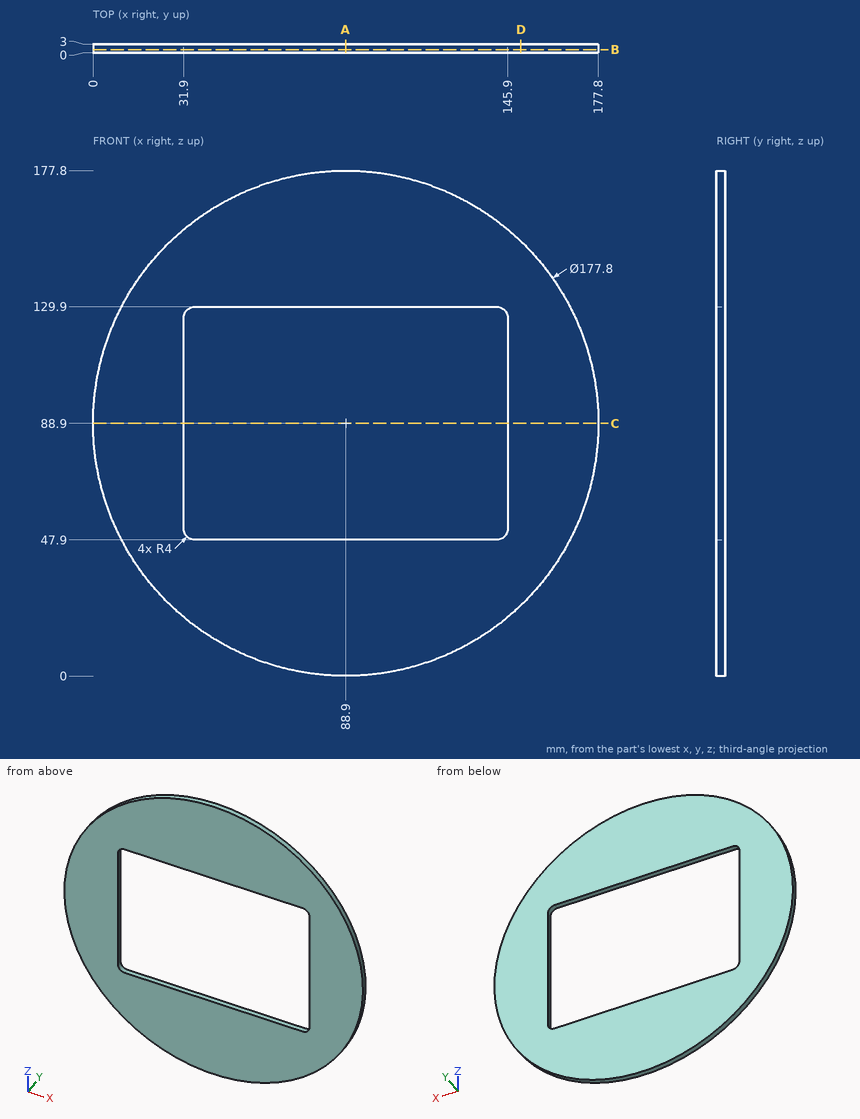
Can you work these out from the drawing? Everything is in mm from the part's minimum corner. Round coordinates to 2 decimals unless told otherwise and drop trailing zeros. Loops run counter-clockwise (first coordinate to the right, second up) from the corner with the lowest first, then second, coordinate; pieces in that order, holes last. Notation, with made-up numbers: (-26.75, 86.25) - (-1.75, 86.25) arc R16 cw to (-1.75, 91.25) - close; hole circle Ø5 at (2, 21). An arc over 180 degrees is marked (long way). Write item = value, one per line. Start each with the question number.
(1) For P1, Ø10, axis at x = 122, z = 124, coming from the +Y side; P2, Ø1.5, axis at y = 2, z = 83.5, coming from the -X side; P3, Ø1.5, axis at y = 1.5, z = 72.5, coming from the +X side; P4, Ø1.5, axis at x = 95, y = 2, coming from the -Z side, each with a flat end and sliding along its axis, tell me the tip position at first contact or that it passes through.
(2) If we section it at D-D (x = 150.5): Please give me the cut outline in (y, z), and give its area (3 significant figures).
(3) If we section it at B-B (y = 1): Please give me the cut outline in (x, z), and give its area (3 significant figures).
(4) If we section it at A-A (x = 88.9): Please give me the cut outline in (y, z), and give its area (3 significant figures).
(5) If we section it at C-C (z = 88.9): Please give me the cut outline in (x, y).
(6) If I drill on probe 1 along Z at (x, y) = (93, 2.6); probe 2 along Z at (x, y) = (91, 0.55); probe 3 along X at (y, z) = (0.3, 66), over which ranges is the centre line in solid material (lowest first)? Write a range as [from, to].
Ans:
q1.P1 = through
q1.P2 = 0.12
q1.P3 = 176.41
q1.P4 = 0.16
q2.outline = (0, 24.8) - (3, 24.8) - (3, 153) - (0, 153) - close
q2.area = 385 mm²
q3.outline = circle Ø177.8 at (88.9, 88.9); hole (31.9, 51.9) arc R4 ccw to (35.9, 47.9) - (141.9, 47.9) arc R4 ccw to (145.9, 51.9) - (145.9, 125.9) arc R4 ccw to (141.9, 129.9) - (35.9, 129.9) arc R4 ccw to (31.9, 125.9) - close
q3.area = 15,500 mm²
q4.outline = (0, 0) - (3, 0) - (3, 47.9) - (0, 47.9) - close; (0, 129.9) - (3, 129.9) - (3, 177.8) - (0, 177.8) - close
q4.area = 287 mm²
q5.outline = (0, 0) - (31.9, 0) - (31.9, 3) - (0, 3) - close; (145.9, 0) - (177.8, 0) - (177.8, 3) - (145.9, 3) - close
q6.probe_1 = [0.09, 47.9], [129.9, 177.71]
q6.probe_2 = [0.02, 47.9], [129.9, 177.78]
q6.probe_3 = [3, 31.9], [145.9, 174.8]
